Input: part model. Units: mm. Frame: model coordinates. Coordinates: 2 decimals unless noted, no trailing zeros. Order: outer loops, then holes, each group sorted by start corner. A loop starts at its lowest first (then second) coordinate and runs counter-clockwise, first axis right, second up. Notation, with made-up numbers: (41, 12) -> (85, 12) arc R32 ccw to (85, 41) -> close; hole circle Ø3 at (36, -35.75). An arc over 180 degrees is marked (long way). Use one line per item in the form item = value. Start each with the question number.
1) Draft query along Y for faces 1 (the cylindrical face through (125.664, 186.205, 1.565)), 2 (the flat face through (75, 285, 3.175)). Return one class per face: pulls with the +Y half, pulls with the -Y half, needs draft (parallel to the pull), parting line crosses it, or undercut.
2) Ray query, line 1 along X through (y, z) = (167, 0.45); line 2 along Y through (x, z) = (26.5, 0.6); line 3 along Y through (x, z) = (49.5, 3). Return the intervals inside material, ascending.
3) Pin query (flat end, axial travel): pin 1 (0.7 mm diameter, centred on x = 35, z = 2, fed in from -Y); pin 2 (1.2 mm diameter, centred on x = 35, z = 2, fed in from +Y); pin 3 (1.2 mm diameter, centred on y = 273.5, z = 1.5, fed in from -X). Return the tip coordinate at first contact, or that it passes through.
4) Section query C-C on z = 2.3. Count the separate pieces of the cut face and the enclosed holes in it, then the cut area to 3 significant figures.
5) Section query A-A on x = 62. Output: boundary loops of the cut face in (y, z) (3 decimals), then the cut area to 3 significant figures.
6) Section query B-B on y = 212. Output: boundary loops of the cut face in (x, z) (3 decimals), then the cut area to 3 significant figures.
from build123d import *

# Parameters (mm, degrees)
SKETCH1_R           = 3.05
SKETCH1_W           = 89.973098966
SKETCH1_H           = 90.646237782
BOSS_EXTRUDE1_DEPTH = 3.175


with BuildPart() as part:
    # Sketch1 → Boss-Extrude1 (new body)
    with BuildSketch(Plane.XY):
        Polygon((0, 308.79500376), (0, 289.867896869), (2.980646754, 289.867896869), (2.980646754, 273.05208143), (9.289682385, 273.05208143), (9.289682385, 274.542404807), (12.717426152, 274.542404807), (12.717426152, 273.05208143), (16.14516992, 273.05208143), (16.14516992, 268.829498528), (12.717426152, 268.829498528), (12.717426152, 267.33917515), (9.289682385, 267.33917515), (9.289682385, 268.829498528), (2.980646754, 268.829498528), (2.980646754, 252.013683088), (0, 252.013683088), (0, 214.159469307), (2.980646754, 214.159469307), (2.980646754, 197.343653867), (9.289682385, 197.343653867), (9.289682385, 198.833977244), (12.717426152, 198.833977244), (12.717426152, 197.343653867), (16.14516992, 197.343653867), (16.14516992, 193.121070965), (12.717426152, 193.121070965), (12.717426152, 191.630747588), (9.289682385, 191.630747588), (9.289682385, 193.121070965), (2.980646754, 193.121070965), (2.980646754, 176.305255525), (0, 176.305255525), (0, 157.378148634), (18.927106891, 157.378148634), (18.927106891, 160.358795389), (35.74292233, 160.358795389), (35.74292233, 166.667831019), (34.252598953, 166.667831019), (34.252598953, 170.095574787), (35.74292233, 170.095574787), (35.74292233, 173.523318554), (39.965505232, 173.523318554), (39.965505232, 170.095574787), (41.45582861, 170.095574787), (41.45582861, 166.667831019), (39.965505232, 166.667831019), (39.965505232, 160.358795389), (56.781320672, 160.358795389), (56.781320672, 157.378148634), (94.635534454, 157.378148634), (94.635534454, 160.358795389), (111.451349893, 160.358795389), (111.451349893, 166.667831019), (109.961026516, 166.667831019), (109.961026516, 170.095574787), (111.451349893, 170.095574787), (111.451349893, 173.523318554), (115.673932795, 173.523318554), (115.673932795, 170.095574787), (117.164256172, 170.095574787), (117.164256172, 166.667831019), (115.673932795, 166.667831019), (115.673932795, 160.358795389), (132.489748235, 160.358795389), (132.489748235, 157.378148634), (151.416855126, 157.378148634), (151.416855126, 176.305255525), (148.436208371, 176.305255525), (148.436208371, 193.121070965), (142.127172741, 193.121070965), (142.127172741, 191.630747588), (138.699428973, 191.630747588), (138.699428973, 193.121070965), (135.271685206, 193.121070965), (135.271685206, 197.343653867), (138.699428973, 197.343653867), (138.699428973, 198.833977244), (142.127172741, 198.833977244), (142.127172741, 197.343653867), (148.436208371, 197.343653867), (148.436208371, 214.159469307), (151.416855126, 214.159469307), (151.416855126, 252.013683088), (148.436208371, 252.013683088), (148.436208371, 268.829498528), (142.127172741, 268.829498528), (142.127172741, 267.33917515), (138.699428973, 267.33917515), (138.699428973, 268.829498528), (135.271685206, 268.829498528), (135.271685206, 273.05208143), (138.699428973, 273.05208143), (138.699428973, 274.542404807), (142.127172741, 274.542404807), (142.127172741, 273.05208143), (148.436208371, 273.05208143), (148.436208371, 289.867896869), (151.416855126, 289.867896869), (151.416855126, 308.79500376), (132.489748235, 308.79500376), (132.489748235, 305.814357006), (115.673932795, 305.814357006), (115.673932795, 299.505321375), (117.164256172, 299.505321375), (117.164256172, 296.077577608), (115.673932795, 296.077577608), (115.673932795, 292.64983384), (111.451349893, 292.64983384), (111.451349893, 296.077577608), (109.961026516, 296.077577608), (109.961026516, 299.505321375), (111.451349893, 299.505321375), (111.451349893, 305.814357006), (94.635534454, 305.814357006), (94.635534454, 308.79500376), (56.781320672, 308.79500376), (56.781320672, 305.814357006), (39.965505232, 305.814357006), (39.965505232, 299.505321375), (41.45582861, 299.505321375), (41.45582861, 296.077577608), (39.965505232, 296.077577608), (39.965505232, 292.64983384), (35.74292233, 292.64983384), (35.74292233, 296.077577608), (34.252598953, 296.077577608), (34.252598953, 299.505321375), (35.74292233, 299.505321375), (35.74292233, 305.814357006), (18.927106891, 305.814357006), (18.927106891, 308.79500376), align=None)
        with Locations((26.087654184, 283.82694987)):
            Circle(SKETCH1_R, mode=Mode.SUBTRACT)
        with Locations(Location((125.873209609, 284.070712088, 0), (0, 0, 180))):
            Circle(SKETCH1_R, mode=Mode.SUBTRACT)
        with Locations((126.06075315, 183.180712088)):
            Circle(SKETCH1_R, mode=Mode.SUBTRACT)
        with Locations(Location((26.27542779, 182.933192277, 0), (0, 0, 180))):
            Circle(SKETCH1_R, mode=Mode.SUBTRACT)
        with Locations((76.074203667, 233.503830979)):
            Rectangle(SKETCH1_W, SKETCH1_H, mode=Mode.SUBTRACT)
    extrude(amount=BOSS_EXTRUDE1_DEPTH)


solid = part.part
Answers below:
q1.face_1 = undercut
q1.face_2 = needs draft
q2.line_1 = 0 to 34.25, 41.46 to 109.96, 117.16 to 151.42
q2.line_2 = 160.36 to 179.89, 185.97 to 280.8, 286.85 to 305.81
q2.line_3 = 160.36 to 188.18, 278.83 to 305.81
q3.pin_1 = 160.36
q3.pin_2 = 305.81
q3.pin_3 = 2.98
q4.separate_pieces = 1
q4.enclosed_holes = 5
q4.area = 13,200 mm^2
q5.outline = (157.378, 0) -> (188.181, 0) -> (188.181, 3.175) -> (157.378, 3.175) -> close; (278.827, 0) -> (308.795, 0) -> (308.795, 3.175) -> (278.827, 3.175) -> close
q5.area = 193 mm^2
q6.outline = (2.981, 0) -> (31.088, 0) -> (31.088, 3.175) -> (2.981, 3.175) -> close; (121.061, 0) -> (148.436, 0) -> (148.436, 3.175) -> (121.061, 3.175) -> close
q6.area = 176 mm^2
